from build123d import *

# Parameters (mm, degrees)
CROQUIS1_W              = 320
CROQUIS1_H              = 40
SALIENTE_EXTRUIR1_DEPTH = 5
CROQUIS2_R              = 2.5
CORTAR_EXTRUIR1_DEPTH   = 5


with BuildPart() as part:
    # Croquis1 → Saliente-Extruir1 (new, symmetric)
    with BuildSketch(Plane.XY):
        Rectangle(CROQUIS1_W, CROQUIS1_H)
    extrude(amount=SALIENTE_EXTRUIR1_DEPTH, both=True)

    # Croquis2 → Cortar-Extruir1 (cut)
    with BuildSketch(Plane.XY):
        with Locations((155, 15)):
            Circle(CROQUIS2_R)
        with Locations((77.5, 15)):
            Circle(CROQUIS2_R)
        with Locations((0, 15)):
            Circle(CROQUIS2_R)
        with Locations((-77.5, 15)):
            Circle(CROQUIS2_R)
        with Locations((-155, 15)):
            Circle(CROQUIS2_R)
        with Locations(Location((155, -15, 0), (0, 0, 180))):
            Circle(CROQUIS2_R)
        with Locations(Location((77.5, -15, 0), (0, 0, 180))):
            Circle(CROQUIS2_R)
        with Locations(Location((0, -15, 0), (0, 0, 180))):
            Circle(CROQUIS2_R)
        with Locations(Location((-77.5, -15, 0), (0, 0, 180))):
            Circle(CROQUIS2_R)
        with Locations(Location((-155, -15, 0), (0, 0, 180))):
            Circle(CROQUIS2_R)
        with Locations((-155, 0)):
            Circle(CROQUIS2_R)
        with Locations(Location((155, 0, 0), (0, 0, 180))):
            Circle(CROQUIS2_R)
    extrude(amount=-CORTAR_EXTRUIR1_DEPTH, mode=Mode.SUBTRACT)


solid = part.part
CAD build for the part. Positions are in the model's coordinates, mm. Give positions to 0.01 mm unless a question says otherwise; leave off trailing zeros. Return JSON: item names as keys, results as strings.
Q1. Mould opens along Y. For faces 1 (the face through (-2, 20, 0)), 2 (the face through (76, 13, -2)), 3 (the face through (-2, 0, -5)), 4 (the face through (-2, -20, 0)) say: pulls with the +Y half, pulls with the -Y half, needs draft (parallel to the pull), parting line crosses it, or undercut.
Working result:
{"face 1": "pulls with the +Y half", "face 2": "undercut", "face 3": "needs draft", "face 4": "pulls with the -Y half"}
Q2. Drill centre lines: line 1 (X direction, y = -15, z = -1.2); line 2 (Y direction, x = 155, z = -1.2); line 3 (Y direction, x = -77.5, z = -3.8). Where is each one in solid material? Low to high.
Working result:
{"line 1": "-160 to -157.5, -152.5 to -80, -75 to -2.5, 2.5 to 75, 80 to 152.5, 157.5 to 160", "line 2": "-20 to -17.5, -12.5 to -2.5, 2.5 to 12.5, 17.5 to 20", "line 3": "-20 to -17.5, -12.5 to 12.5, 17.5 to 20"}
Q3. Flat gauge pin, fed straight in: pin 1 (1.5 mm diameter, centred on x = -155.5, y = 0, fed in from -Z). Where does the tip first touch, or does it go through?
Working result:
{"pin 1": "z = 0"}
